Could you check a few things on this model? Use its own coordinates, in mm. Face numbers are marked on the shaded views. A direction names the side the tool comes from. Round coordinates to 2 decimals unless told otherwise and drop trailing zeros. Loops run counter-clockwise (first coordinate to the right, second up) from the corner with the lowest first, then second, coordinate; pieces in that order, holes last. Notation, with made-up numbers: (-33.75, -21.5) -> (-10.75, -21.5) arc R28 ccw to (-10.75, 8.5) -> close; hole circle Ø9 at (-24, 28.25). An arc over 180 degrees is marked (long way). One line per item, written item: value.
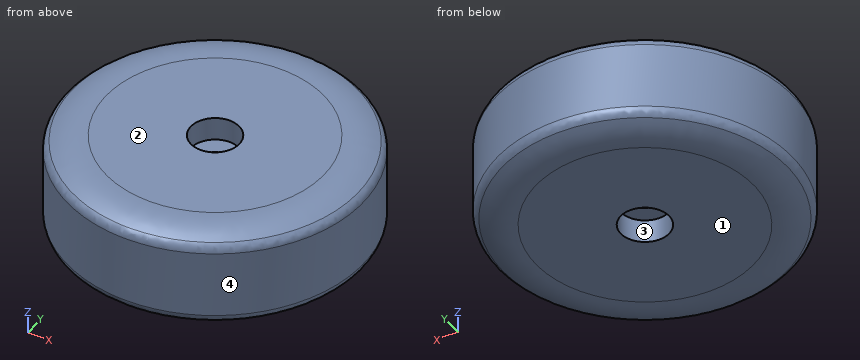
```python
from build123d import *

# Parameters (mm, degrees)
F2_R     = 3.55
F3_DEPTH = 50.1686232636
F2_R_2   = 12.5
F4_DEPTH = 12
F5_START = -38
F5_DEPTH = 12
F6_R     = 5


with BuildPart() as f1:
    # F0 (on Right) → F1 (revolve)
    with BuildSketch(Plane.YZ):
        with BuildLine():
            Line((-56.2, 0), (0, 0))
            Line((0, 0), (0, 50))
            Line((0, 50), (-56.2, 50))
            ThreePointArc((-56.2, 50), (-66.642974542, 49.2718981679), (-76.2, 45))
            Line((-76.2, 45), (-76.2, 5))
            ThreePointArc((-76.2, 5), (-66.642974542, 0.7281018321), (-56.2, 0))
        make_face()
    revolve(axis=Axis((0, 0, 25), (0, 0, 1)))

    # F2 (on face) → F3 (cut, through all)
    with BuildSketch(Plane.XY.offset(50)):
        Circle(F2_R)
    extrude(amount=-F3_DEPTH, mode=Mode.SUBTRACT)

    # F2 (on face) → F4 (cut)
    with BuildSketch(Plane.XY.offset(50)):
        Circle(F2_R_2)
        Polygon((-6.9282032303, 0), (-3.4641016151, 6), (3.4641016151, 6), (6.9282032303, 0), (3.4641016151, -6), (-3.4641016151, -6), align=None, mode=Mode.SUBTRACT)
        Polygon((3.4641016151, 6), (-3.4641016151, 6), (-6.9282032303, 0), (-3.4641016151, -6), (3.4641016151, -6), (6.9282032303, 0), align=None)
        Circle(F2_R, mode=Mode.SUBTRACT)
    extrude(amount=-F4_DEPTH, mode=Mode.SUBTRACT)

    # F2 (on face) → F5 (cut)
    with BuildSketch(Plane.XY.offset(50).offset(F5_START)):
        Circle(F2_R_2)
        Polygon((-6.9282032303, 0), (-3.4641016151, 6), (3.4641016151, 6), (6.9282032303, 0), (3.4641016151, -6), (-3.4641016151, -6), align=None, mode=Mode.SUBTRACT)
        Polygon((3.4641016151, 6), (-3.4641016151, 6), (-6.9282032303, 0), (-3.4641016151, -6), (3.4641016151, -6), (6.9282032303, 0), align=None)
        Circle(F2_R, mode=Mode.SUBTRACT)
    extrude(amount=-F5_DEPTH, mode=Mode.SUBTRACT)

    # F6
    f6_edges = [f1.edges().sort_by_distance(p)[0] for p in [
        (0, 76.2, 45),
        (0, 76.2, 5),
    ]]
    fillet(f6_edges, radius=F6_R)


solid = f1.part
```
(1) We'd pull the mould along X, two halves only. Please class the marked faces 3 and 4: +X half, -X half, draft (parallel to the pull), parting line (faces both ways), or undercut.
Results below:
face 3: undercut
face 4: parting line
(2) On a 3-axis mill with a long thin cutter (end or side, diameter ignored), from which of +Z, -Z, +X, -X, +Y, -Y can I reach the whole of each face in a straight line? I mean the marked faces 1 and 2. Say none if no direction works.
Results below:
face 1: -Z
face 2: +Z
(3) For pin 1 Ø5 at (x, y) = (27.5, 8.5) entering from -Z; pin 2 Ø5 at (x, z) = (50, 32) entering from +Y; pin 3 Ø9 at (x, y) = (0, 0) entering from +Z, each with a flat end and sliding along its axis, tell me the tip position at first contact or that it passes through.
Results below:
pin 1: stops at z = 0
pin 2: stops at y = 59.58
pin 3: stops at z = 38
(4) Please list where these lines run through material, in increasing order: L1, parallel to Y at x = 0, z = 40.75; L2, parallel to Y at x = 0, z = 19; L3, parallel to Z at x = -37, y = -11.
Results below:
L1: y = -76.2 to -12.5, 12.5 to 76.2
L2: y = -76.2 to -3.55, 3.55 to 76.2
L3: z = 0 to 50
(5) Imagine slicing it at A-A on z = 30. Write out the boundary of the cut face in (x, y), then the cut area to 3 significant figures.
Results below:
outline: circle Ø152.4 at (0, 0); hole circle Ø7.1 at (0, 0)
area: 18,200 mm²
